For this review, use the dimensioned drawing (mm, ordinates from the lowest corner) and the shaded views. A direction names the side the tool comes from. Coordinates: 2 decimals unless noted, no trailing zeros. Order: outer loops, then holes, each group sorted by start corner. A loop starts at its lowest first (then second) coordinate and runs counter-clockwise, first axis right, second up. Notation, with made-up numbers: (-12.5, 12.5) -> (33.5, 12.5) arc R22 ccw to (33.5, 30.5) -> close; hole circle Ø5 at (78.25, 58). An arc over 180 degrees is marked (long way). Use one line per item in the form item = value. Start each with the question number.
(1) Take a section at D-D (y = 7.5). State the section outline as (x, z) points, then the cut area to 3 significant figures.
(2) For the marked faces 1, 2, 3, 4 and 5, list the 3-axis set-ups (+Z, -Z, +X, -X, +Y, -Y) from which the entire face can be reached by the end or side of a thin tool; tool diameter is ignored.
(3) Insertion check: pin 1 Ø6 at (x, y) = (3.5, 19.5) entering from +Z; pin 2 Ø1.5 at (y, z) = (15.5, 2.5) entering from -X; pin 3 Ø6 at (x, y) = (2.5, 11) entering from -Z. Each pin has a flat end and moves straight along its axis. Give the tip position at first contact, or say it passes through.
(4) Take a section at B-B (y = 21.25). State the section outline as (x, z) points, then the cut area to 3 significant figures.
(5) Take a section at A-A (y = 25.95). State the section outline as (x, z) points, then the cut area to 3 significant figures.
(6) Take a section at C-C (y = 13.25). State the section outline as (x, z) points, then the cut area to 3 significant figures.
(7) Wall thickness on line 1 along Y through (x, z) = (5.6, 5); line 2 along Y through (x, z) = (8.5, 7.25); line 3 along X through (y, z) = (25, 7): over which ranges is each line inside the solid? List them lowest first.
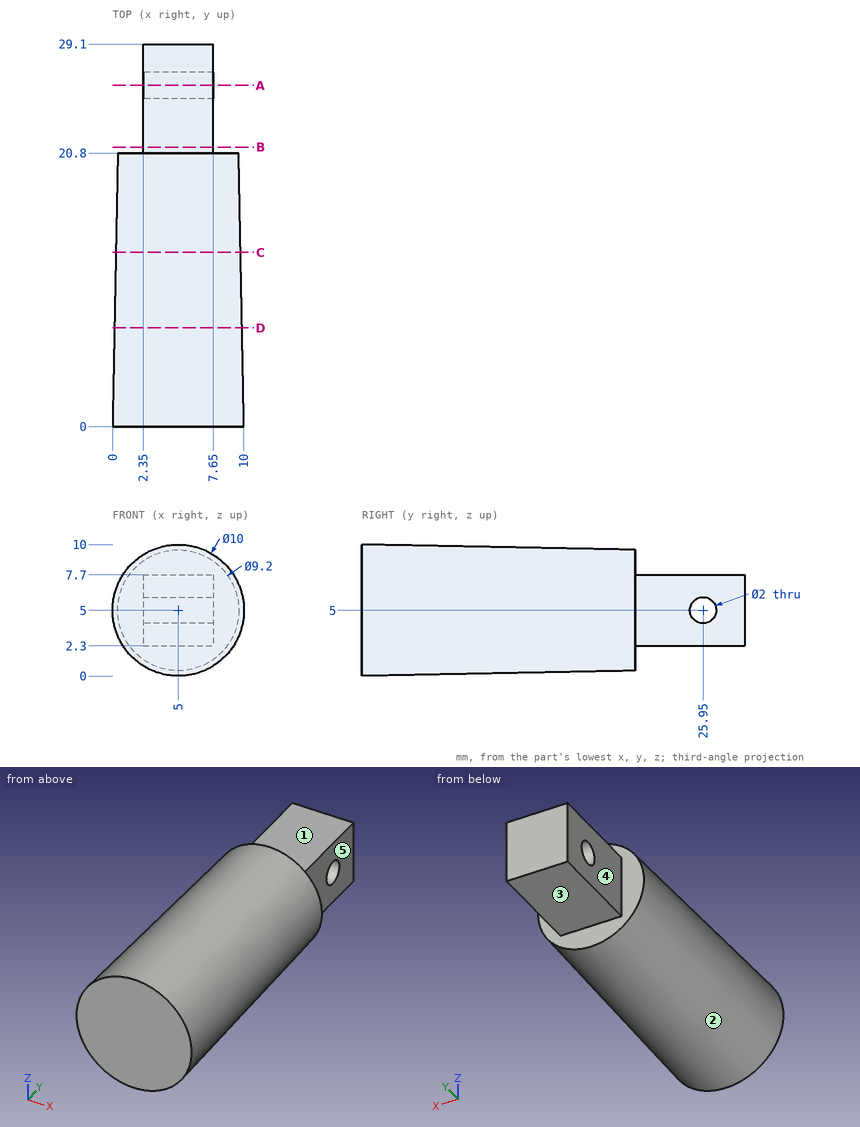
Findings:
q1.outline = circle Ø9.71 at (5, 5)
q1.area = 74.1 mm²
q2.face_1 = +Z, +X, -X, +Y
q2.face_2 = +Y
q2.face_3 = -Z, +X, -X, +Y
q2.face_4 = +Z, -Z, -X, +Y
q2.face_5 = +Z, -Z, +X, +Y
q3.pin_1 = 9.68
q3.pin_2 = 0.64
q3.pin_3 = 0.18
q4.outline = (2.35, 2.3) -> (7.65, 2.3) -> (7.65, 7.7) -> (2.35, 7.7) -> close
q4.area = 28.6 mm²
q5.outline = (2.35, 2.3) -> (7.65, 2.3) -> (7.65, 4) -> (2.35, 4) -> close; (2.35, 6) -> (7.65, 6) -> (7.65, 7.7) -> (2.35, 7.7) -> close
q5.area = 18.0 mm²
q6.outline = circle Ø9.49 at (5, 5)
q6.area = 70.7 mm²
q7.line_1 = 0 to 24.95, 26.95 to 29.1
q7.line_2 = 0 to 20.8
q7.line_3 = 2.35 to 7.65
